```python
from build123d import *

# Parameters (mm, degrees)
BOSS_EXTRUDE1_DEPTH = 5
CUT_EXTRUDE1_DEPTH  = 95.158544522
SKETCH6_R           = 7.25
BOSS_EXTRUDE3_DEPTH = 15
SKETCH3_R           = 5.25
CUT_EXTRUDE2_DEPTH  = 20
SKETCH5_R           = 1.5
CUT_EXTRUDE3_DEPTH  = 5
CUT_EXTRUDE4_START  = -2.5
SKETCH8_R           = 11
SKETCH8_R_2         = 7.25
CUT_EXTRUDE4_DEPTH  = 2.5


with BuildPart() as part:
    # Sketch1 → Boss-Extrude1 (new body)
    with BuildSketch(Plane.XY):
        Polygon((-30.995, 36.381727213), (-14, 67.5), (14, 67.5), (30.995, 36.381727213), (14.995, 8.668914292), (15, 8.660254038), (15.005, 8.651593784), (47.005, 8.651593784), (65.456714755, -21.625644347), (51.456714755, -45.874355653), (16.01, -45.033320997), (0.01, -17.320508076), (0, -17.320508076), (-0.01, -17.320508076), (-16.01, -45.033320997), (-51.456714755, -45.874355653), (-65.456714755, -21.625644347), (-47.005, 8.651593784), (-15.005, 8.651593784), (-15, 8.660254038), (-14.995, 8.668914292), align=None)
    extrude(amount=BOSS_EXTRUDE1_DEPTH)

    # Sketch2 → Cut-Extrude1 (cut, through all)
    with BuildSketch(Plane.XY.offset(5)):
        Polygon((-28.872149716, 2.651593784), (-12.118974925, -26.293867874), (-19.521225678, -39.114942267), (-48.040387098, -39.791608731), (-58.480737567, -21.708391269), (-43.63514651, 2.651593784), align=None)
        Polygon((-24.113920832, 36.463348484), (-16.71167008, 23.64227409), (16.732422435, 23.678218224), (24.113920832, 36.463348484), (10.440350469, 61.5), (-10.440350469, 61.5), align=None)
        Polygon((43.63514651, 2.651593784), (28.830645005, 2.651593784), (12.139727281, -26.329812008), (19.521225678, -39.114942267), (48.040387098, -39.791608731), (58.480737567, -21.708391269), align=None)
    extrude(amount=-CUT_EXTRUDE1_DEPTH, mode=Mode.SUBTRACT)

    # Sketch6 → Boss-Extrude3 (add)
    with BuildSketch(Plane(origin=(0, 0, 0), x_dir=(-1, 0, 0), z_dir=(0, 0, -1))):
        with Locations(Location((0, 0, 0), (0, 0, 180))):
            Circle(SKETCH6_R)
    extrude(amount=BOSS_EXTRUDE3_DEPTH)

    # Sketch3 → Cut-Extrude2 (cut)
    with BuildSketch(Plane(origin=(0, 0, -15), x_dir=(-1, 0, 0), z_dir=(0, 0, -1))):
        Circle(SKETCH3_R)
    extrude(amount=-CUT_EXTRUDE2_DEPTH, mode=Mode.SUBTRACT)

    # Sketch5 → Cut-Extrude3 (cut)
    with BuildSketch(Plane.XY.offset(5)):
        with Locations((-45.443044798, 5.870544436)):
            Circle(SKETCH5_R)
        with Locations((-62.08538883, -21.665632507)):
            Circle(SKETCH5_R)
        with Locations((-49.805684066, -42.93470506)):
            Circle(SKETCH5_R)
        with Locations((-17.637483295, -42.290100822)):
            Circle(SKETCH5_R)
        with Locations((27.80556106, 36.419560852)):
            Circle(SKETCH5_R)
        with Locations((12.279704321, 64.600342034)):
            Circle(SKETCH5_R)
        with Locations((-12.279705207, 64.600342034)):
            Circle(SKETCH5_R)
        with Locations((-27.805561947, 36.419560852)):
            Circle(SKETCH5_R)
        with Locations((17.637482409, -42.290100822)):
            Circle(SKETCH5_R)
        with Locations((49.80568318, -42.93470506)):
            Circle(SKETCH5_R)
        with Locations((62.085387944, -21.665632507)):
            Circle(SKETCH5_R)
        with Locations((45.443043912, 5.870544436)):
            Circle(SKETCH5_R)
    extrude(amount=-CUT_EXTRUDE3_DEPTH, mode=Mode.SUBTRACT)

    # Sketch8 → Cut-Extrude4 (cut)
    with BuildSketch(Plane(origin=(0, 0, 0), x_dir=(-1, 0, 0), z_dir=(0, 0, -1)).offset(CUT_EXTRUDE4_START)):
        Circle(SKETCH8_R)
        Circle(SKETCH8_R_2, mode=Mode.SUBTRACT)
    extrude(amount=CUT_EXTRUDE4_DEPTH, mode=Mode.SUBTRACT)


solid = part.part
```
Model file for the job. Use its own axes, mm. A direction names the side the tool comes from. Coordinates: 2 decimals unless noted, no trailing zeros. Loops run counter-clockwise (first coordinate to the right, second up) from the corner with the lowest first, then second, coordinate; pieces in that order, holes last. Notation, with made-up numbers: (45.5, 32) - (49.5, 32) arc R10 ccw to (49.5, 43) - close; hole circle Ø6 at (27.25, -16.5). An arc over 180 degrees is marked (long way). Write item = value, one per line. Start each with the question number.
Item 1: 3-axis set-ups, long thin cutter, end or side, ignore diameter. For faces 5 (the face through (-51.162, -9.699, 2.535)), 6 (the face through (-22.88, 22.33, 2.46)), 7 (the face through (2.38, -10.74, 1.27)): which of +Z, -Z, +X, -X, +Y, -Y reach the whole face in a straight line?
Item 2: Saw through at A-A, the plane y = 44.5. List the corners of the cut face in (x, z).
Item 3: Saw through at C-C, the plane y = 0. List the corners of the cut face in (x, z).
Item 4: Saw through at D-D, the plane z = -6. List the corners of the cut face in (x, y).
Item 5: Pull direction X, two halves, no side cores. Call faces 1 (the face through (8.12, -31.37, 2.46)), 2 (the face through (31, 8.652, 2)), 3 (the face through (56.102, -6.275, 2.465)), 4 (the face through (20.37, 29.98, 2.54)): +X half, -X half, draft (parallel to the pull), parting line (faces both ways), or undercut.
Item 6: Saw through at B-B, the plane x = -57. List the corners of the cut face in (y, z), then the cut area to 3 significant figures.
Item 7: Wall check: probe 1 along Y at (x, z) = (0, 1.65); probe 2 along X at (y, z) = (-8, 1.5); probe 3 along Z at (x, y) = (-25.5, 44.5). Give the ranges that are in metal, low to high. Write a range as [from, to].
Item 8: Drop flat-ended pins along their axis: pin 1 Ø2.5 at (x, y) = (-27.81, 36.42) entering from +Z; pin 2 Ø5.5 at (x, z) = (31, 2) entering from +Y; pin 3 Ø2.5 at (x, z) = (-34.5, 1.5) entering from -Y; pin 4 Ø8 at (y, z) = (-5, -10.5) entering from -X. Give the stop position or say it passes through.
Answers:
q1.face_5 = +Z, -Z
q1.face_6 = +Z, -Z, -X
q1.face_7 = -Z
q2.outline = (-26.56, 0) - (-19.72, 0) - (-19.72, 5) - (-26.56, 5) - close; (19.72, 0) - (26.56, 0) - (26.56, 5) - (19.72, 5) - close
q3.outline = (-52.28, 0) - (-45.25, 0) - (-45.25, 5) - (-52.28, 5) - close; (-27.34, 0) - (-11, 0) - (-11, 2.5) - (-7.25, 2.5) - (-7.25, -15) - (-5.25, -15) - (-5.25, 5) - (-27.34, 5) - close; (5.25, -15) - (7.25, -15) - (7.25, 2.5) - (11, 2.5) - (11, 0) - (27.3, 0) - (27.3, 5) - (5.25, 5) - close; (45.25, 0) - (52.28, 0) - (52.28, 5) - (45.25, 5) - close
q4.outline = circle Ø14.5 at (0, 0); hole circle Ø10.5 at (0, 0)
q5.face_1 = undercut
q5.face_2 = draft
q5.face_3 = +X half
q5.face_4 = undercut
q6.outline = (-36.27, 0) - (-24.27, 0) - (-24.27, 5) - (-36.27, 5) - close; (-19.28, 0) - (-7.75, 0) - (-7.75, 5) - (-19.28, 5) - close
q6.area = 118 mm2
q7.probe_1 = [-17.32, -11], [-7.25, -5.25], [5.25, 7.25], [11, 23.66], [61.5, 67.5]
q7.probe_2 = [-57.15, -50.13], [-22.71, -7.55], [7.55, 22.7], [50.13, 57.15]
q7.probe_3 = [0, 5]
q8.pin_1 = through
q8.pin_2 = 41.41
q8.pin_3 = -45.5
q8.pin_4 = -7.18
